For this review, take the finished solid that the model builds, in its own axes (mm). A direction names the side the tool comes from. Give positions to 0.01 mm unless a question says otherwise; leave off trailing zeros. Write each loop counter-clockwise with the first axis right and the second up, starting at its lowest first coordinate (ties: lowest second). Pieces come first, ordered by that corner, then holes.
from build123d import *

# Parameters (mm, degrees)
F2_W           = 17
F2_H           = 12
F3_DEPTH       = 25
F5_D           = 2.4
F5_DEPTH       = 12
F5_CBORE_D     = 4.4
F5_CBORE_DEPTH = 2
F5_TIP         = 0.7210327428


# Not quite as in the source:
# - the program builds the solid bodies; features that only make, move or delete a surface that nothing else refers to are left out


with BuildPart() as f3:
    # F2 (on Top) → F3 (new body)
    with BuildSketch(Plane.XY):
        with Locations((0, 16)):
            Rectangle(F2_W, F2_H)
    extrude(amount=F3_DEPTH)

    # F5
    with Locations(Plane.XZ.offset(-10)):
        with Locations((-3.9957389235, 18.5837522149), (0, 21.3394463062), (0, 13.3731160313), (4.3110894039, 8.4640979767), (-4.0247985162, 5.713914521)):
            CounterBoreHole(F5_D / 2, F5_CBORE_D / 2, F5_CBORE_DEPTH, depth=F5_DEPTH)
            with Locations((0, 0, -(F5_DEPTH + F5_TIP / 2))):  # 118° drill point
                Cone(0, F5_D / 2, F5_TIP, mode=Mode.SUBTRACT)


solid = f3.part
(1) We need section A-A (x = 0). Write out the cut boundary in (y, z).
(2) Clearance check with a flat-ended pin moving along its axis: pin 1 Ø3 at (x, z) = (0, 13.37) entering from -Y. State where the tip first meets the part, or that it passes through.
(3) We need section D-D (z = 6). Write out the cut boundary in (x, y), and give its area (3 significant figures).
(4) For L1, parallel to Z at x = 0, y = 16; L2, parallel to Z at x = 0, y = 10.75; L3, parallel to X at y = 21.5, z = 5.75, list the stretches that pass through material, from the lowest coordinate up.
(5) The part is to be moulded in two halves that separate along Z. For faces 1 (the flat face through (0, 16, 25)), 2 (the flat face through (-2, 10, 12)), 3 (the cylindrical face through (-2.826, 17.07, 5.767)), say which applies: +Z half, -Z half, draft (parallel to the pull), parting line (faces both ways), or undercut.
(6) We need section C-C (x = 4.75). Write out the cut boundary in (y, z).
(7) Tool access review of faces 4 (the cylindrical face through (-1.926, 10.986, 6.375)), 5 (the flat face through (2, 22, 12)): name each direction out of +Z, -Z, +X, -X, +Y, -Y from which nothing blocks a thin tool from reaching the whole face with its end or side.
(8) We need section B-B (y = 18.5). Write out the cut boundary in (x, z).
The answers:
1. outline: (10, 0) - (22, 0) - (22, 12.17) - (12, 12.17) - (12, 11.17) - (10, 11.17) - close; (10, 15.57) - (12, 15.57) - (12, 14.57) - (22, 14.57) - (22, 20.14) - (12, 20.14) - (12, 19.14) - (10, 19.14) - close; (10, 23.54) - (12, 23.54) - (12, 22.54) - (22, 22.54) - (22, 25) - (10, 25) - close
2. pin 1: stops at y = 12
3. outline: (-8.5, 10) - (-6.21, 10) - (-6.21, 12) - (-5.19, 12) - (-5.19, 22) - (-8.5, 22) - close; (-2.86, 12) - (-1.84, 12) - (-1.84, 10) - (8.5, 10) - (8.5, 22) - (-2.86, 22) - close
3. area: 172 mm2
4. L1: z = 0 to 12.17, 14.57 to 20.14, 22.54 to 25
4. L2: z = 0 to 11.17, 15.57 to 19.14, 23.54 to 25
4. L3: x = -8.5 to -5.22, -2.83 to 8.5
5. face 1: +Z half
5. face 2: draft
5. face 3: undercut
6. outline: (10, 0) - (22, 0) - (22, 7.35) - (12, 7.35) - (12, 6.31) - (10, 6.31) - close; (10, 10.62) - (12, 10.62) - (12, 9.58) - (22, 9.58) - (22, 25) - (10, 25) - close
7. face 4: -Y
7. face 5: +Z, -Z, +X, -X, +Y
8. outline: (-8.5, 0) - (8.5, 0) - (8.5, 25) - (-8.5, 25) - close; hole circle Ø2.4 at (-4.02, 5.71); hole circle Ø2.4 at (-4, 18.58); hole circle Ø2.4 at (0, 13.37); hole circle Ø2.4 at (0, 21.34); hole circle Ø2.4 at (4.31, 8.46)
